Autodesk Inventor part; units mm, degrees
ref_plane "YZ Plane" through (0, 0, 0) normal (1, 0, 0) x (0, 1, 0)
ref_plane "XZ Plane" through (0, 0, 0) normal (0, 1, 0) x (-1, 0, 0)
ref_plane "XY Plane" through (0, 0, 0) normal (0, 0, 1) x (1, 0, 0)
sketch "スケッチ1" plane through (0, 0, 0) normal (0, 0, 1) x (1, 0, 0)
  line L0 (0, 25) -> (-4.25, 25)
  line L1 (-4.25, 25) -> (-4.25, 0)
  line L2 (-4.25, 0) -> (0, 0)
  line L3 (0, 0) -> (0, 25)
  line L4 (0, -5) -> (0, 30)
  line L5 (-5.1, 0) -> (0.85, 0)
  dimension "d2" = 4.25
  dimension "d3" = 25
revolve "回転1" add sketch "スケッチ1" angle 360 about axis through (0, -10, 0) along (0, 1, 0)
sketch "スケッチ3" plane through (0, 25, 0) normal (0, 1, 0) x (1, 0, 0)
  circle A0 centre (0, 0) radius 3
  dimension "d5" = 6
extrude "押し出し1" cut sketch "スケッチ3" against normal blind 5
sketch "スケッチ4" plane through (0, 0, 0) normal (0, -1, 0) x (1, 0, 0)
  circle A0 centre (0, 0) radius 4.25
  line L0 (4.25, 3.25) -> (6.25, 3.25)
  line L1 (4.25, -3.25) -> (6.25, -3.25)
  line L2 (6.25, -3.25) -> (6.25, 3.25)
  line L3 (3.4369, 2.5) -> (4.25, 2.5)
  line L4 (-6.15, 0) -> (7.15, 0)
  line L5 (4.25, 3.25) -> (4.25, 2.5)
  line L6 (4.25, 0) -> (4.25, -3.25)
  line L7 (3.4369, -2.5) -> (4.25, -2.5)
  dimension "d9" = 6.5
  dimension "d10" = 2
  dimension "d11" = 2.5
  dimension "d12" = 5
extrude "押し出し2" add sketch "スケッチ4" against normal blind 20 contours L6 L7 A0 | A0 L3 L5 L0 L2 L4 | L4 L2 L1 L6
fillet "フィレット1" radius 0.5 4 edges at (6.25, 10, 3.25) (6.25, 10, -3.25) (4.25, 10, -3.25) (4.25, 10, 3.25)
properties part number "flat_cover_6mm"
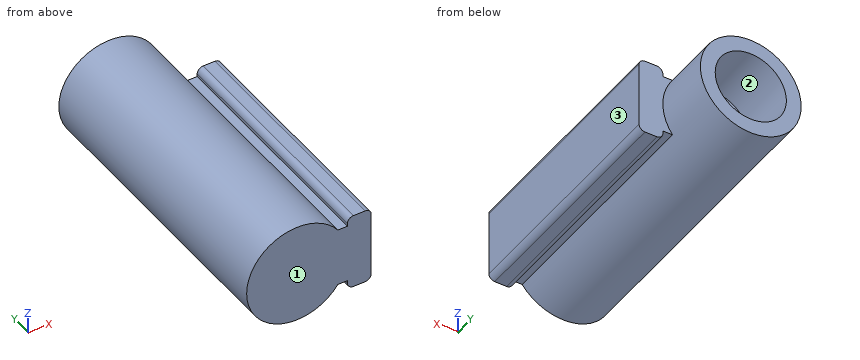
Verification items for the finished model (mm, model axes). Face numbers are marked on the shaded views. Coordinates: 2 decimals unless noted, no trailing zeros. Order: outer loops, then holes, each group sorted by start corner. A loop starts at its lowest first (then second) coordinate and runs counter-clockwise, first axis right, second up. Notation, with made-up numbers: (12, 54) -> (61, 54) arc R25 cw to (61, 82) -> close; hole circle Ø5 at (70, 73). An arc over 180 degrees is marked (long way). Put each result on its own line as item: value. Start each with the question number.
1. Cross-section at B-B, the plane z = 0. Record the boundary of the cut face in (x, y), then the cut area to 4 significant figures.
2. Cross-section at C-C, the plane y = 10. Record the boundary of the cut face in (x, z), then the cut area to 3 significant figures.
3. Material ranges on L1, parallel to X at y = 21.95, z = 0; L2, parallel to Y at x = 5, z = 1.5, recorded low to high. Write a range as [from, to].
4. Cross-section at A-A, the plane x = 0. Record the boundary of the cut face in (y, z).
5. Cross-section at D-D, the plane x = 4. Record the boundary of the cut face in (y, z).
6. Go/stop test with flat-tipped pins: pin 1 Ø0.9 at (x, y) = (4, 11.5) entering from +Z; pin 2 Ø1.5 at (x, y) = (2, 13.5) entering from -Z; pin 3 Ø0.8 at (x, y) = (5, 10) entering from -Z. Record where each tip stops, or that it passes through.
7. Mould release check, pull along X, two halves, no side actions. Record for the marked faces 1, 2 and 3: released by +X, released by -X, zero draft, split by the parting line, or undercut.
Computed:
1. outline: (-4.25, 0) -> (6.25, 0) -> (6.25, 20) -> (4.25, 20) -> (4.25, 25) -> (3, 25) -> (3, 20) -> (-3, 20) -> (-3, 25) -> (-4.25, 25) -> close
1. area: 222.5 mm2
2. outline: (3.44, -2.5) -> (4.25, -2.5) -> (4.25, -2.75) arc R0.5 ccw to (4.75, -3.25) -> (5.75, -3.25) arc R0.5 ccw to (6.25, -2.75) -> (6.25, 2.75) arc R0.5 ccw to (5.75, 3.25) -> (4.75, 3.25) arc R0.5 ccw to (4.25, 2.75) -> (4.25, 2.5) -> (3.44, 2.5) arc R4.25 ccw (long way) to start
2. area: 70.8 mm2
3. L1: [-4.25, -3], [3, 4.25]
3. L2: [0, 20]
4. outline: (0, -4.25) -> (25, -4.25) -> (25, -3) -> (20, -3) -> (20, 3) -> (25, 3) -> (25, 4.25) -> (0, 4.25) -> close
5. outline: (0, -2.5) -> (20, -2.5) -> (20, -1.44) -> (25, -1.44) -> (25, 1.44) -> (20, 1.44) -> (20, 2.5) -> (0, 2.5) -> close
6. pin 1: z = 3.15
6. pin 2: z = -4.06
6. pin 3: z = -3.25
7. face 1: zero draft
7. face 2: undercut
7. face 3: released by +X
